Work out the finished part from the listing and answer in its coordinate system (mm). A direction names the side the tool comes from. Coordinates: 2 decimals unless noted, no trailing zeros. Order: outer loops, then holes, each group sorted by start corner. A loop starts at its lowest first (then second) coordinate and runs counter-clockwise, first axis right, second up. Notation, with made-up numbers: M -8,51.5 L 22,51.5 A15 ccw 22,74.5 Z; hole C 7,42.5 d4. An arc over 180 degrees is marked long. Write item = value, one per line. Start each with the question number.
Q1. Find section B-B on x = -27. Give the vertices of the cut face in (y, z).
Q2. Straight lines are drawn through the part: line 1 along X through (y, z) = (-0.5, 6) (3 decimals); line 2 along X through (y, z) = (0, -15.5); line 3 along X through (y, z) = (-43, 18). For each, find the intervals that lie inside material, in ascending order.
Q3. Find section A-A on z = 1. Give the vertices of the cut face in (x, y), and give its area (3 significant figures).
Q4. A tool of negligible diameter and unlimited length cuts with its end or side. For faces 4 (the flat face through (0, -9, -29.074)), 5 (the flat face through (-22, -30, 0)), 6 (the flat face through (-3, -3, 0)), 7 (the flat face through (-18, 0, 30)), 8 (the flat face through (9, 9, 29.074)), from which of +Z, -Z, +X, -X, +Y, -Y can it reach the whole face along a straight path? Write none if from no direction.
Q5. Determine the mould class of faces 1 (the cylindrical face through (4.032, 6.324, -2.872)), 2 (the cylindrical face through (-20.28, -49.4, 47.43)), 3 (the flat face through (-36, -25, 24)) for opening direction X: released by +X, released by -X, zero draft, split by the parting line, or undercut.
Q6. Find section C-C on z = -15.5. Give the vertices of the cut face in (x, y), and give its area (3 significant figures).
Q7. Each of these flat-tipped pins is pushed along its axis until it touches: P1, Ø18, axis at x = -9.5, y = -29.5, coming from the -Z side; P2, Ø3, axis at x = -9, z = 27, coming from the +Y side; P3, Ø2, axis at x = -11, z = 21.5, coming from the +Y side. Where does it stop, or does it pass through?
```python
from build123d import *

# Parameters (mm, degrees)
F0_R     = 25
F0_R_2   = 7.5
F1_DEPTH = 29.07393
F2_W     = 36
F2_H     = 48
F3_DEPTH = 50
F4_SIZE  = 5
F5_R     = 5
F6_R     = 2
F7_R     = 5


with BuildPart() as f1:
    # F0 (on Top) → F1 (new body, symmetric)
    with BuildSketch(Plane.XY):
        Circle(F0_R)
        Circle(F0_R_2, mode=Mode.SUBTRACT)
    extrude(amount=F1_DEPTH, both=True)

    # F2 (on Front) → F3 (join)
    with BuildSketch(Plane.XZ):
        with Locations((-18, 24)):
            Rectangle(F2_W, F2_H)
    extrude(amount=F3_DEPTH)

    # F4
    f4_edges = [f1.edges().sort_by_distance(p)[0] for p in [
        (0, 25, 29.07393),
        (0, 7.5, 29.07393),
    ]]
    chamfer(f4_edges, length=F4_SIZE)

    # F5
    f5_edges = [f1.edges().sort_by_distance(p)[0] for p in [
        (0, -25, 48),
    ]]
    fillet(f5_edges, radius=F5_R)

    # F6
    f6_edges = [f1.edges().sort_by_distance(p)[0] for p in [
        (-20.5, -50, 48),
    ]]
    fillet(f6_edges, radius=F6_R)

    # F7
    f7_edges = [f1.edges().sort_by_distance(p)[0] for p in [
        (-25, 0, -29.07393),
    ]]
    fillet(f7_edges, radius=F7_R)


solid = f1.part
```
Findings below:
q1.outline = M -50,0 L 0,0 L 0,48 L -48,48 A2 ccw -50,46 Z
q2.line_1 = -36 to 0, 7.483 to 24.995
q2.line_2 = -25 to -7.5, 7.5 to 25
q2.line_3 = -36 to 0
q3.outline = M -36,-50 L -2,-50 A2 ccw 0,-48 L 0,-25 A25 ccw long -25,0 L -36,0 Z; hole M -7.5,0 L 0,0 L 0,-7.5 A7.5 ccw long Z
q3.area = 3,140 mm^2
q4.face_4 = -Z, +X, -X, +Y, -Y
q4.face_5 = -Z, -X, -Y
q4.face_6 = -Z
q4.face_7 = +Z
q4.face_8 = +Z, +X, +Y
q5.face_1 = undercut
q5.face_2 = zero draft
q5.face_3 = released by -X
q6.outline = C 0,0 d50; hole C 0,0 d15
q6.area = 1,790 mm^2
q7.P1 = -28.66
q7.P2 = 21.9
q7.P3 = 22.91
